For this review, take the finished solid that the model builds, in its own axes (mm). Give positions to 0.01 mm unless a question says otherwise; leave off trailing zeros. Order: outer loops, then holes, each group sorted by start corner. A loop starts at its lowest first (then second) coordinate and runs counter-clockwise, first axis right, second up.
Autodesk Inventor part; units mm, degrees
ref_plane "YZ Plane" through (0, 0, 0) normal (1, 0, 0) x (0, 1, 0)
ref_plane "XZ Plane" through (0, 0, 0) normal (0, 1, 0) x (-1, 0, 0)
ref_plane "XY Plane" through (0, 0, 0) normal (0, 0, 1) x (1, 0, 0)
sketch "Schizzo1" plane through (0, 0, 0) normal (0, 0, 1) x (1, 0, 0)
  line L0 (75, -65) -> (75, 65)
  line L1 (65, 75) -> (-75, 75)
  line L2 (-85, 65) -> (-85, -65)
  line L3 (-75, -75) -> (65, -75)
  arc A0 (-85, -65) -> (-75, -75) centre (-75, -65) ccw
  arc A1 (-75, 75) -> (-85, 65) centre (-75, 65) ccw
  arc A2 (75, 65) -> (65, 75) centre (65, 65) ccw
  arc A3 (65, -75) -> (75, -65) centre (65, -65) ccw
  circle A4 centre (-81, 48) radius 2
  circle A5 centre (-81, -48) radius 2
  circle A6 centre (71, 48) radius 2
  circle A7 centre (71, -48) radius 2
  circle A8 centre (-58, -71) radius 2
  circle A9 centre (-58, 71) radius 2
  circle A10 centre (48, 71) radius 2
  circle A11 centre (48, -71) radius 2
  dimension "d32" = 10
  dimension "d42" = 4
  dimension "d43" = 4
  dimension "d45" = 4
  dimension "d46" = 4
  dimension "d53" = 4
  dimension "d54" = 4
  dimension "d55" = 4
  dimension "d56" = 4
extrude "Estrusione2" add sketch "Schizzo1" along normal blind 9
sketch "Schizzo2" plane through (0, 0, 0) normal (0, 0, -1) x (-1, 0, 0)
  line L0 (75, -65) -> (75, 65)
  line L1 (65, 75) -> (-75, 75)
  line L2 (-85, 65) -> (-85, -65)
  line L3 (-75, -75) -> (65, -75)
  circle A0 centre (0, -36) radius 2
  circle A1 centre (0, 36) radius 2
  circle A2 centre (55, -36) radius 2
  circle A3 centre (55, 36) radius 2
  circle A4 centre (-75, -36) radius 2
  circle A5 centre (-75, 36) radius 2
  arc A6 (-85, -65) -> (-75, -75) centre (-75, -65) ccw
  arc A7 (-75, 75) -> (-85, 65) centre (-75, 65) ccw
  arc A8 (75, 65) -> (65, 75) centre (65, 65) ccw
  arc A9 (65, -75) -> (75, -65) centre (65, -65) ccw
  line L4 (-25, -20) -> (-25, -20)
  line L5 (-20, -15) -> (-20, 15)
  line L6 (-25, 20) -> (-25, 20)
  line L7 (-30, 15) -> (-30, -15)
  arc A10 (-30, -15) -> (-25, -20) centre (-25, -15) ccw
  arc A11 (-25, -20) -> (-20, -15) centre (-25, -15) ccw
  arc A12 (-20, 15) -> (-25, 20) centre (-25, 15) ccw
  arc A13 (-25, 20) -> (-30, 15) centre (-25, 15) ccw
  point P0 (0, 0)
  point P1 (0, 0)
  point P2 (-25, 0)
  dimension "d64" = 4
  dimension "d65" = 4
  dimension "d66" = 4
  dimension "d67" = 4
  dimension "d68" = 4
  dimension "d69" = 4
  dimension "d70" = 10
  dimension "d71" = 5
move or copy body "Sposta corpo1" bodies to move or copy 1 copy no translate (10, 0, 0)
extrude "Estrusione3" cut sketch "Schizzo2" against normal blind 9 contours A11 A10 L7 A13 A12 L5
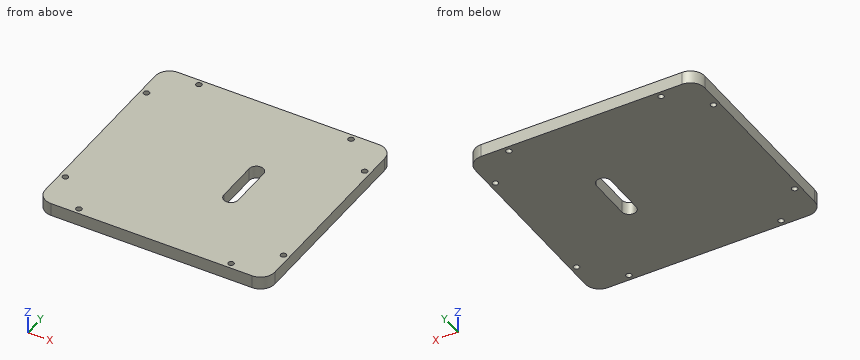
1) We need section B-B on x = 58. Give the boundary of the cut face in (y, z), then the cut area to 3 significant figures.
Answer sheet:
outline: (-75, 0) - (-73, 0) - (-73, 9) - (-75, 9) - close; (-69, 0) - (69, 0) - (69, 9) - (-69, 9) - close; (73, 0) - (75, 0) - (75, 9) - (73, 9) - close
area: 1,280 mm2
2) We need section C-C on z = 7.5. Count the separate pieces of the cut face and the enclosed holes in it, then the cut area to 3 significant figures.
Answer sheet:
separate pieces: 1
enclosed holes: 9
area: 23,400 mm2
3) To check wall thickness, follow line 1 (Y direction, x = -71, z = 5.75); line 2 (Y direction, x = -48, z = 6.25); line 3 (X direction, y = -11, z = 7). State the ranges of each line that lie inside material, in increasing order.
Answer sheet:
line 1: y = -73 to -50, -46 to 46, 50 to 73
line 2: y = -75 to -73, -69 to 69, 73 to 75
line 3: x = -75 to 20, 30 to 85
4) We need section D-D on y = -17.5. Give the boundary of the cut face in (x, z), then the cut area to 3 significant figures.
Answer sheet:
outline: (-75, 0) - (20.67, 0) - (20.67, 9) - (-75, 9) - close; (29.33, 0) - (85, 0) - (85, 9) - (29.33, 9) - close
area: 1,360 mm2
5) We need section A-A on y = -48. Give the boundary of the cut face in (x, z).
Answer sheet:
outline: (-75, 0) - (-73, 0) - (-73, 9) - (-75, 9) - close; (-69, 0) - (79, 0) - (79, 9) - (-69, 9) - close; (83, 0) - (85, 0) - (85, 9) - (83, 9) - close
